```python
from build123d import *

# Parameters (mm, degrees)
SKETCH_1_W             = 80
SKETCH_1_H             = 26
EXTRUDE_1_DEPTH        = 34
HOLE_WIZARD_M6_1_D     = 5
HOLE_WIZARD_M6_1_DEPTH = 15
HOLE_WIZARD_M6_1_TIP   = 1.502151548
HOLE_WIZARD_M6_2_D     = 5
HOLE_WIZARD_M6_2_DEPTH = 15
HOLE_WIZARD_M6_2_TIP   = 1.502151548


with BuildPart() as part:
    # 草图1 → 凸台-拉伸1 (new body)
    with BuildSketch(Plane.XY):
        with Locations((40, 13)):
            Rectangle(SKETCH_1_W, SKETCH_1_H)
    extrude(amount=EXTRUDE_1_DEPTH)

    # M6 螺纹孔1
    with Locations(Plane.XY.offset(34)):
        with Locations((70, 21), (70, 5), (30, 21), (30, 5)):
            Hole(HOLE_WIZARD_M6_1_D / 2, depth=HOLE_WIZARD_M6_1_DEPTH)
            with Locations((0, 0, -(HOLE_WIZARD_M6_1_DEPTH + HOLE_WIZARD_M6_1_TIP / 2))):  # 118° drill point
                Cone(0, HOLE_WIZARD_M6_1_D / 2, HOLE_WIZARD_M6_1_TIP, mode=Mode.SUBTRACT)

    # M6 螺纹孔2
    with Locations(Plane(origin=(0, 0, 0), x_dir=(-1, 0, 0), z_dir=(0, 0, -1))):
        with Locations((-10, 5), (-10, 21), (-70, 21), (-70, 5)):
            Hole(HOLE_WIZARD_M6_2_D / 2, depth=HOLE_WIZARD_M6_2_DEPTH)
            with Locations((0, 0, -(HOLE_WIZARD_M6_2_DEPTH + HOLE_WIZARD_M6_2_TIP / 2))):  # 118° drill point
                Cone(0, HOLE_WIZARD_M6_2_D / 2, HOLE_WIZARD_M6_2_TIP, mode=Mode.SUBTRACT)


solid = part.part
```
Design review of the part built by this model. Coordinates are the model's own, in mm. A direction names the side the tool comes from. Coordinates: 2 decimals unless noted, no trailing zeros. Order: outer loops, then holes, each group sorted by start corner. A loop starts at its lowest first (then second) coordinate and runs counter-clockwise, first axis right, second up.
1) Clearance check with flat-ended pins moving along their axes: pin 1 (8 mm diameter, centred on x = 30, y = 21, fed in from +Z); pin 2 (4 mm diameter, centred on x = 70, y = 21, fed in from +Z); pin 3 (4 mm diameter, centred on x = 70, y = 5, fed in from -Z); pin 4 (4.5 mm diameter, centred on x = 70, y = 21, fed in from +Z). State where each tip first meets the part, or that it passes through.
2) Mouldability with a two-part tool opening along Y and no side actions: class faces 4 (the flat face through (39, 26, 17)), 5 (the flat face through (80, 13, 17)), 6 (the conical face through (30.4, 20.83, 17.76)) as +Y half, -Y half, draft (parallel to the pull), parting line (faces both ways), or undercut.
3) Wall thickness on line 1 along X through (y, z) = (21, 10.5); line 2 along Y through (x, z) = (70, 6.75); line 3 along X through (y, z) = (21, 22.5): over which ranges is each line inside the solid? List them lowest first.
4) For faces 1 (the cylindrical face through (30.33, 23.48, 26.4)), 2 (the cylindrical face through (9.67, 7.48, 7.6)), 3 (the flat face through (39, 0, 17)), list the 3-axis set-ups (+Z, -Z, +X, -X, +Y, -Y) from which the entire face can be reached by the end or side of a thin tool; tool diameter is ignored.
5) Take a section at A-A, the plane z = 20.5. Give the boundary of the cut face in (x, y), and give its area (3 significant figures).
Returned:
1. pin 1: stops at z = 34
1. pin 2: stops at z = 18.7
1. pin 3: stops at z = 15.3
1. pin 4: stops at z = 18.85
2. face 4: +Y half
2. face 5: draft
2. face 6: undercut
3. line 1: x = 0 to 7.5, 12.5 to 67.5, 72.5 to 80
3. line 2: y = 0 to 2.5, 7.5 to 18.5, 23.5 to 26
3. line 3: x = 0 to 27.5, 32.5 to 67.5, 72.5 to 80
4. face 1: +Z
4. face 2: -Z
4. face 3: +Z, -Z, +X, -X, -Y
5. outline: (0, 0) - (80, 0) - (80, 26) - (0, 26) - close; hole circle Ø5 at (30, 5); hole circle Ø5 at (30, 21); hole circle Ø5 at (70, 5); hole circle Ø5 at (70, 21)
5. area: 2,000 mm2
